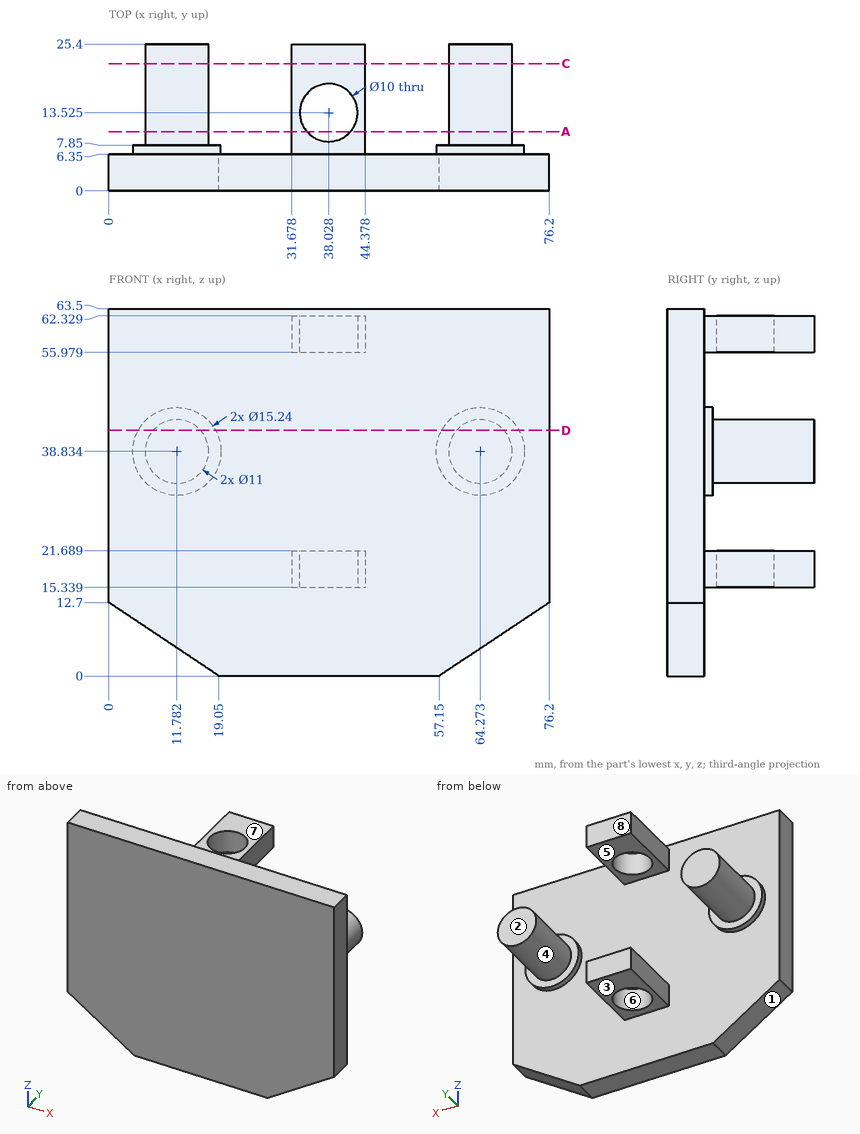
The drawing under review shows one solid part. Ordinate dimensions are in mm from its lowest x, y, z. A direction names the side the tool comes from. Round coordinates to 2 decimals unless told otherwise and drop trailing zeros. Write each loop counter-clockwise with the first axis right and the second up, starting at its lowest first coordinate (ties: lowest second). Pieces come first, ordered by that corner, then holes. Notation, with made-up numbers: M 6.5,-21 L 35.5,-21 A17 ccw 35.5,9 Z; hole C -15.5,51 d7. An arc over 180 degrees is marked long. One line per item, written item: value. Start each with the question number.
(1) Insertion check: pin 1 (3 mm diameter, centred on y = 12.5, z = 59.5, fed in from -X); pin 2 (3 mm diameter, centred on y = 12, z = 57.5, fed in from +X); pin 3 (10 mm diameter, centred on x = 36.5, y = 13.5, fed in from -Z); pin 4 (2 mm diameter, centred on x = 60, z = 13.5, fed in from -Y). Each pin has a flat end and moves straight along its axis. Give the tip position at first contact, or say it passes through.
(2) Wall thickness on line 1 (Z direction, x = 34, y = 8); line 2 (Y direction, x = 70, z = 46.5); line 3 (Y direction, x = 6, z = 37): over which ranges is each line inside the solid? List them lowest first.
(3) We need section D-D (z = 42.5). Give the boundary of the cut face in (x, y).
(4) We need section C-C (y = 22). Give the boundary of the cut face in (x, z).
(5) The part is to be moulded in two halves that separate along Y. For the marked faces 6, 7 and 8, say which applies: released by +Y, released by -Y, zero draft, split by the parting line, or undercut.
(6) Machinability: for the marked faces 1, 2, 3, 4 and 5, which of the approach directions +Z, -Z, +X, -X, +Y, -Y give a long, thin tool a straight path to every point of the face, cutting with its end or side? Answer none if there is none.
(7) We need section A-A (y = 10.25). Give the boundary of the cut face in (x, z), and give its area (3 significant figures).
Result:
1. pin 1: x = 31.68
1. pin 2: x = 44.38
1. pin 3: z = 15.34
1. pin 4: y = 0
2. line 1: 15.34 to 21.69, 55.98 to 62.33
2. line 2: 0 to 6.35
2. line 3: 0 to 7.85
3. outline: M 0,0 L 76.2,0 L 76.2,6.35 L 70.95,6.35 L 70.95,7.85 L 68.37,7.85 L 68.37,25.4 L 60.17,25.4 L 60.17,7.85 L 57.59,7.85 L 57.59,6.35 L 18.46,6.35 L 18.46,7.85 L 15.88,7.85 L 15.88,25.4 L 7.68,25.4 L 7.68,7.85 L 5.1,7.85 L 5.1,6.35 L 0,6.35 Z
4. outline: C 11.78,38.83 d11; M 31.68,15.34 L 44.38,15.34 L 44.38,21.69 L 31.68,21.69 Z; M 31.68,55.98 L 44.38,55.98 L 44.38,62.33 L 31.68,62.33 Z; C 64.27,38.83 d11
5. face 6: undercut
5. face 7: zero draft
5. face 8: released by +Y
6. face 1: -Z, -X, +Y, -Y
6. face 2: +Z, -Z, +X, -X, +Y
6. face 3: -Z, +X, -X, +Y
6. face 4: +Y
6. face 5: +X, -X, +Y
7. outline: C 11.78,38.83 d11; M 31.68,15.34 L 34.25,15.34 L 34.25,21.69 L 31.68,21.69 Z; M 31.68,55.98 L 34.25,55.98 L 34.25,62.33 L 31.68,62.33 Z; M 41.81,15.34 L 44.38,15.34 L 44.38,21.69 L 41.81,21.69 Z; M 41.81,55.98 L 44.38,55.98 L 44.38,62.33 L 41.81,62.33 Z; C 64.27,38.83 d11
7. area: 255 mm²
